```python
from build123d import *

# Parameters (mm, degrees)
F0_W     = 14.5715866238
F0_H     = 6.5456330776
F0_W_2   = 4.949297756
F0_W_3   = 5.8135613799
F0_H_2   = 2.0267963409
F0_W_4   = 3.5245139152
F0_H_3   = 21.7774156481
F1_DEPTH = 25.4


with BuildPart() as f1:
    # F0 (on Top) → F1 (new body)
    with BuildSketch(Plane.XY):
        Polygon((-33.7974205613, 48.0205528438), (-49.6319867671, 48.0205528438), (-49.6319867671, 30.4928608239), (-44.5602796972, 30.4928608239), (-44.5602796972, 32.5196571648), (-38.7467183173, 32.5196571648), (-38.7467183173, 39.0652902424), (-33.7974205613, 39.0652902424), align=None)
        with Locations((-26.5116272494, 35.7924737036)):
            Rectangle(F0_W, F0_H)
        with Locations((-36.2720694393, 35.7924737036)):
            Rectangle(F0_W_2, F0_H)
        with Locations((-41.6534990072, 31.5062589943)):
            Rectangle(F0_W_3, F0_H_2)
        Polygon((-38.7467183173, 30.4928608239), (-44.5602796972, 30.4928608239), (-44.5602796972, 0), (30.7543519884, 0), (30.7543519884, 10.7422415167), (30.7543519884, 32.5196571648), (-19.2258339375, 32.5196571648), (-19.2258339375, 9.3785366043), (-38.7467183173, 9.3785366043), align=None)
        Polygon((-19.2258339375, 32.5196571648), (-33.7974205613, 32.5196571648), (-33.7974205613, 30.4928608239), (-38.7467183173, 30.4928608239), (-38.7467183173, 9.3785366043), (-19.2258339375, 9.3785366043), align=None)
        with Locations((32.516608946, 21.6309493408)):
            Rectangle(F0_W_4, F0_H_3)
    extrude(amount=-F1_DEPTH)


solid = f1.part
```
Input: part model. Units: mm. Frame: model coordinates. A direction names the side the tool comes from. Give positions to 0.01 mm unless a question says otherwise; leave off trailing zeros. Loops run counter-clockwise (first coordinate to the right, second up) from the corner with the lowest first, then second, coordinate; pieces in that order, holes last. Notation, with made-up numbers: (-32, 4) -> (1, 4) arc R21 cw to (1, 10) -> close; hole circle Ø4 at (-25, -8). An arc over 180 degrees is marked (long way). Use a Markdown table: item, result.
Q1. Pull-direction query (Y, two-part tool) for faces 6 (the flat face through (-47, 30.493, -13)), 7 (the flat face through (-36, 30.493, -13)), 8 (the flat face through (-19.226, 36, -13)); classes: pulls with the +Y half, pulls with the -Y half, needs draft (parallel to the pull), parting line crosses it, or undercut.
Entries:
| item | result |
|---|---|
| face 6 | pulls with the -Y half |
| face 7 | undercut |
| face 8 | needs draft |
Q2. Access query for faces 1 (the flat face through (32, 10.742, -13)), 2 (the flat face through (-44.56, 15, -13)), 3 (the flat face through (-42, 48.021, -13)), 4 (the flat face through (-38.747, 31, -13)), 5 (the flat face through (8, 32.52, -13)). Directions: +Z, -Z, +X, -X, +Y, -Y. A direction counts if a zero-diameter tool reaches every point of the face in a straight line with its end or side. Return the directions, or none.
Entries:
| item | result |
|---|---|
| face 1 | +Z, -Z, +X, -Y |
| face 2 | +Z, -Z, -X, -Y |
| face 3 | +Z, -Z, +X, -X, +Y |
| face 4 | +Z, -Z |
| face 5 | +Z, -Z, +X, +Y |
Q3. Section query C-C, the plane x = 14.5. Return the cut outline in (y, z), plus the area to 3 significant figures.
Entries:
| item | result |
|---|---|
| outline | (0, -25.4) -> (32.52, -25.4) -> (32.52, 0) -> (0, 0) -> close |
| area | 826 mm² |
Q4. Section query A-A, the plane z = -14.25. Return the cut outline in (x, y).
Entries:
| item | result |
|---|---|
| outline | (-49.63, 30.49) -> (-44.56, 30.49) -> (-44.56, 0) -> (30.75, 0) -> (30.75, 10.74) -> (34.28, 10.74) -> (34.28, 32.52) -> (-19.23, 32.52) -> (-19.23, 39.07) -> (-33.8, 39.07) -> (-33.8, 48.02) -> (-49.63, 48.02) -> close; hole (-38.75, 30.49) -> (-33.8, 30.49) -> (-33.8, 32.52) -> (-38.75, 32.52) -> close |
Q5. First-contact query: P1, Ø3, axis at y = 22, z = -4.5, coming from the -X side; P2, Ø12, axis at y = 7.5, z = -7, coming from the +X side; P3, Ø4.5, axis at y = 41.5, z = -6.5, coming from the +X side; P4, Ø1.5, axis at x = -46, z = -7.5, coming from the -Y side. Flat tips, straight axial feed; report the tip coordinate or a pass-through.
Entries:
| item | result |
|---|---|
| P1 | stops at x = -44.56 |
| P2 | stops at x = 34.28 |
| P3 | stops at x = -33.8 |
| P4 | stops at y = 30.49 |
Q6. Ray query, probe 1 along X at (y, z) = (31.5, -21.5); probe 2 along Y at (x, z) = (-22.5, -16.75); probe 3 along X at (y, z) = (19, -7). Return the intervals inside material, ascending. Write a range as from..to.
Entries:
| item | result |
|---|---|
| probe 1 | x = -49.63..-38.75, -33.8..34.28 |
| probe 2 | y = 0..39.07 |
| probe 3 | x = -44.56..34.28 |
Q7. Section query B-B, the plane y = 42. Return the cut outline in (x, z), plus the area to 3 significant figures.
Entries:
| item | result |
|---|---|
| outline | (-49.63, -25.4) -> (-33.8, -25.4) -> (-33.8, 0) -> (-49.63, 0) -> close |
| area | 402 mm² |
